```python
from build123d import *

# Parameters (mm, degrees)
ESBO_O1_R                = 6.125
RESSALTO_EXTRUS_O1_DEPTH = 22
ESBO_O2_OUTSIDE_W        = 72
ESBO_O2_OUTSIDE_H        = 63
ESBO_O2_OUTSIDE_R        = 10
CORTE_EXTRUS_O1_DEPTH    = 1.5
ESBO_O3_OUTSIDE_W        = 72
ESBO_O3_OUTSIDE_H        = 63
ESBO_O3_OUTSIDE_R        = 10
CORTE_EXTRUS_O2_DEPTH    = 1.5


with BuildPart() as part:
    # Esboço1 → Ressalto-extrusão1 (new body)
    with BuildSketch(Plane.XY):
        with BuildLine():
            ThreePointArc((-30.781182975, -21.553216354), (-31.830295908, -22.369078713), (-33, -23))
            Line((-33, -23), (-53, -23))
            Line((-53, -23), (-55, -21))
            Line((-55, -21), (-53, -19))
            Line((-53, -19), (-45.812043902, -16.114839283))
            ThreePointArc((-45.812043902, -16.114839283), (-43.50890364, -13.67237999), (-43.877574187, -10.335593438))
            ThreePointArc((-43.877574187, -10.335593438), (-46.755205534, 0), (-43.877574187, 10.335593438))
            ThreePointArc((-43.877574187, 10.335593438), (-43.50890364, 13.67237999), (-45.812043902, 16.114839283))
            Line((-45.812043902, 16.114839283), (-53, 19))
            Line((-53, 19), (-55, 21))
            Line((-55, 21), (-53, 23))
            Line((-53, 23), (-33, 23))
            ThreePointArc((-33, 23), (-30.448735361, 22.582285193), (-28.163895976, 21.372762185))
            Line((-28.163895976, 21.372762185), (0, 0))
            Line((0, 0), (-30.781182975, -21.553216354))
        make_face()
        with Locations((-23, 0)):
            Circle(ESBO_O1_R, mode=Mode.SUBTRACT)
    extrude(amount=RESSALTO_EXTRUS_O1_DEPTH)

    # Esboço2 outside → Corte-extrusão1 (cut)
    with BuildSketch(Plane.XY.offset(22)):
        with Locations((-27.5, 0)):
            Rectangle(ESBO_O2_OUTSIDE_W, ESBO_O2_OUTSIDE_H)
        with Locations((-23, 0)):
            Circle(ESBO_O2_OUTSIDE_R, mode=Mode.SUBTRACT)
    extrude(amount=-CORTE_EXTRUS_O1_DEPTH, mode=Mode.SUBTRACT)

    # Esboço3 outside → Corte-extrusão2 (cut)
    with BuildSketch(Plane(origin=(0, 0, 0), x_dir=(-1, 0, 0), z_dir=(0, 0, -1))):
        with Locations((27.5, 0)):
            Rectangle(ESBO_O3_OUTSIDE_W, ESBO_O3_OUTSIDE_H)
        with Locations(Location((23, 0, 0), (0, 0, 180))):
            Circle(ESBO_O3_OUTSIDE_R, mode=Mode.SUBTRACT)
    extrude(amount=-CORTE_EXTRUS_O2_DEPTH, mode=Mode.SUBTRACT)


solid = part.part
```
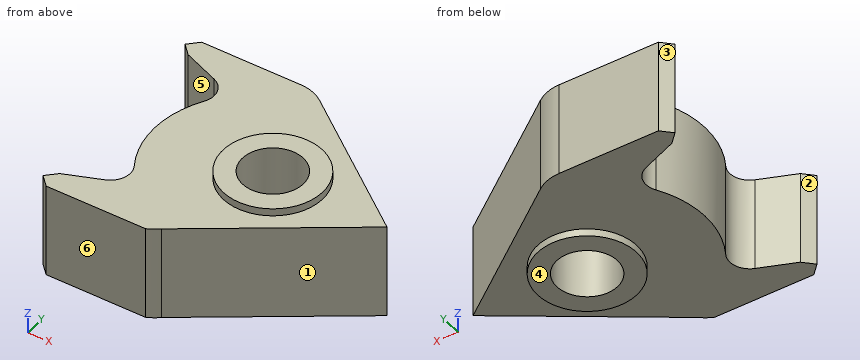
Can you work these out from the model? Positions are in its coordinate system, mm. Face numbers are marked on the shaded views. A direction names the side the tool comes from. Give positions to 0.01 mm unless a question says otherwise; leave off trailing zeros. Loops run counter-clockwise (first coordinate to the right, second up) from the corner with the lowest first, then second, coordinate; pieces in that order, holes last. Notation, with made-up numbers: M -16.75,52 L 32.25,52 A29 cw 32.25,78 Z; hole C 46,42.5 d1. An arc over 180 degrees is marked long. One line per question, with ' | ' between items. Start each with the question number.
Q1. If we section it at D-D (x = -48.5): Please give me the cut outline in (y, z), plus the area to 3 significant figures.
Q2. If we section it at A-A (z = 2.75): Please give me the cut outline in (x, y) (3 decimals), plus the area to 3 significant figures.
Q3. If we mould it in two halves opening along Y, with no side actions, what happens to the marked faces 3, 4, 5 and 6? For each: +Y half, -Y half, draft (parallel to the pull), parting line (faces both ways), or undercut.
Q4. For the marked faces 1 and 2, which set-ups out of +Z, -Z, +X, -X, +Y, -Y let a thin tool reach every point of the face, with its end or its side?
Q5. If we section it at B-B (x = -18): Please give me the cut outline in (y, z), plus the area to 3 significant figures.
Q6. For pin 1 Ø6 at (x, y) = (-44, -17.5) entering from -Z; pin 2 Ø5 at (y, z) = (9.5, 2.5) entering from -X; pin 3 Ø7.5 at (x, y) = (-23, 0) entering from -Z; pin 4 Ø8 at (x, y) = (-38.5, -8.5) entering from +Z, each with a flat end and sliding along its axis, tell me the tip position at first contact or that it passes through.
Q7. If we section it at C-C (y = -7.5): Please give me the cut outline in (x, z), plus the area to 3 significant figures.
Q8. If I drill on line 1 (Z direction, x = -10, y = -5); line 2 (Y direction, x = -23, z = 8.25) (3 decimals); line 3 (X direction, y = 3, z = 3.5), over which ranges is the centre line in solid material (lowest first)? Write a range as from..to.
Computed:
1) outline: M -23,1.5 L -17.19,1.5 L -17.19,20.5 L -23,20.5 Z; M 17.19,1.5 L 23,1.5 L 23,20.5 L 17.19,20.5 Z | area: 221 mm²
2) outline: M -55,-21 L -53,-23 L -33,-23 A8 ccw -30.781,-21.553 L 0,0 L -28.164,21.373 A8 ccw -33,23 L -53,23 L -55,21 L -53,19 L -45.812,16.115 A4 cw -43.878,10.336 A20 ccw -43.878,-10.336 A4 cw -45.812,-16.115 L -53,-19 Z; hole C -23,0 d12.25 | area: 1,330 mm²
3) face 3: +Y half | face 4: draft | face 5: undercut | face 6: -Y half
4) face 1: +Z, -Z, +X, -Y | face 2: +Z, -Z, -X
5) outline: M -12.6,1.5 L -8.66,1.5 L -8.66,0 L -3.54,0 L -3.54,22 L -8.66,22 L -8.66,20.5 L -12.6,20.5 Z; M 3.54,0 L 8.66,0 L 8.66,1.5 L 13.66,1.5 L 13.66,20.5 L 8.66,20.5 L 8.66,22 L 3.54,22 Z | area: 395 mm²
6) pin 1: stops at z = 1.5 | pin 2: stops at x = -45.49 | pin 3: passes through | pin 4: stops at z = 20.5
7) outline: M -45.3,1.5 L -29.61,1.5 L -29.61,0 L -16.39,0 L -16.39,1.5 L -10.71,1.5 L -10.71,20.5 L -16.39,20.5 L -16.39,22 L -29.61,22 L -29.61,20.5 L -45.3,20.5 Z | area: 697 mm²
8) line 1: z = 1.5..20.5 | line 2: y = -16.105..-6.125, 6.125..17.454 | line 3: x = -46.53..-28.34, -17.66..-3.95
